```python
from build123d import *

# Parameters (mm, degrees)
F1_DEPTH = 1.5875


with BuildPart() as f1:
    # F0 (on Front) → F1 (new body)
    with BuildSketch(Plane.XZ):
        with BuildLine():
            Line((-2.835184, -45.032743), (-2.835184, -91.849111))
            Line((-2.835184, -91.849111), (43.704942, -115.692325))
            ThreePointArc((43.704942, -115.692325), (49.329511, -117.777947), (55.286339, -118.486325))
            Line((55.286339, -118.486325), (101.152416, -118.486325))
            ThreePointArc((101.152416, -118.486325), (112.176016, -68.440927), (101.152416, -18.39553))
            Line((101.152416, -18.39553), (55.286339, -18.39553))
            ThreePointArc((55.286339, -18.39553), (49.329511, -19.103907), (43.704942, -21.18953))
            Line((43.704942, -21.18953), (-2.835184, -45.032743))
        make_face()
    extrude(amount=F1_DEPTH)


solid = f1.part
```
Verification items for the finished model (mm, model axes). Coordinates: 2 decimals unless noted, no trailing zeros. Write each loop counter-clockwise with the first axis right and the second up, starting at its lowest first coordinate (ties: lowest second). Pieces come first, ordered by that corner, then holes. Notation, with made-up numbers: (85.5, -12.75) - (105.5, -12.75) arc R21 cw to (105.5, 15.25) - close; hole circle Ø2 at (-36.75, 72). An arc over 180 degrees is marked (long way). Write item = value, one per line.
Q1. Cross-section at C-C (x = 105). Enter the section's corners in (y, z).
Answer:
outline = (-1.59, -109.16) - (0, -109.16) - (0, -27.72) - (-1.59, -27.72) - close
Q2. Material ranges on L1, parallel to X at y = -0.7, z = -69.5; L2, parallel to Z at x = 3, y = -0.85; L3, parallel to Z at x = 8.5, y = -0.3, recorded low to high. Write a range as from..to.
Answer:
L1 = -2.84..112.17
L2 = -94.84..-42.04
L3 = -97.66..-39.23
Q3. Cross-section at B-B (z = -112). Enter the section's corners in (x, y).
Answer:
outline = (36.5, -1.59) - (103.93, -1.59) - (103.93, 0) - (36.5, 0) - close
Q4. Cross-section at A-A (y = -0.5). Enter the section's corners in (x, z), plus the area to 3 significant figures.
Answer:
outline = (-2.84, -91.85) - (43.7, -115.69) arc R25.4 ccw to (55.29, -118.49) - (101.15, -118.49) arc R119.11 ccw to (101.15, -18.4) - (55.29, -18.4) arc R25.4 ccw to (43.7, -21.19) - (-2.84, -45.03) - close
area = 9,760 mm²
Q5. Go/stop test with a flat-tipped pin: pin 1 Ø10 at (x, z) = (41, -85) entering from +Y. Record where the tip stops, or that it passes through.
Answer:
pin_1 = 0
